Geometry: final body of the model. Coordinates: model frame, mm. A direction names the side the tool comes from. Give positions to 0.01 mm unless a question says otherwise; leave off trailing zeros. Write each loop counter-clockwise with the first axis right and the second up, starting at its lowest first coordinate (ties: lowest second). Pieces come first, ordered by that corner, then holes. Notation, with made-up numbers: M 73.5,18.25 L 109.5,18.25 A23 ccw 109.5,44.25 Z; hole C 5,-10.75 d6. An arc over 180 degrees is marked long. Answer as a JSON object with one key per item and string values.
from build123d import *

# Parameters (mm, degrees)
SKETCH_1_W          = 15.5
SKETCH_1_H          = 8
EXTRUDE_1_DEPTH     = 72
SKETCH_2_W          = 12.7
SKETCH_2_H          = 2
CUT_EXTRUDE_1_DEPTH = 75.082724032
SKETCH_3_W          = 15.5
SKETCH_3_H          = 4
EXTRUDE_2_DEPTH     = 2
SKETCH_5_R          = 2.1
CUT_EXTRUDE_3_DEPTH = 10


with BuildPart() as part:
    # 草图1 → 凸台-拉伸1 (new body)
    with BuildSketch(Plane.XY):
        with Locations((7.75, 4)):
            Rectangle(SKETCH_1_W, SKETCH_1_H)
    extrude(amount=EXTRUDE_1_DEPTH)

    # 草图2 → 切除-拉伸1 (cut, through all)
    with BuildSketch(Plane(origin=(0, 0, 0), x_dir=(-1, 0, 0), z_dir=(0, 0, -1))):
        with Locations((-7.75, 1)):
            Rectangle(SKETCH_2_W, SKETCH_2_H)
    extrude(amount=-CUT_EXTRUDE_1_DEPTH, mode=Mode.SUBTRACT)

    # 草图3 → 凸台-拉伸2 (add)
    with BuildSketch(Plane(origin=(0, 8, 0), x_dir=(1, 0, 0), z_dir=(0, 1, 0))):
        with Locations((7.75, -70)):
            Rectangle(SKETCH_3_W, SKETCH_3_H)
    extrude(amount=EXTRUDE_2_DEPTH)

    # 草图5 → 切除-拉伸3 (cut)
    with BuildSketch(Plane.XY.offset(72)):
        with Locations((3.75, 5)):
            Circle(SKETCH_5_R)
        with Locations(Location((11.75, 5, 0), (0, 0, 180))):
            Circle(SKETCH_5_R)
    extrude(amount=-CUT_EXTRUDE_3_DEPTH, mode=Mode.SUBTRACT)


solid = part.part
1) Pull-direction query (Y, two-part tool) for faces 1 (the flat face through (4, 5, 62)), 2 (the flat face through (15, 0, 35)), 3 (the flat face through (8, 10, 70)), 4 (the flat face through (1.4, 1, 35)); classes: pulls with the +Y half, pulls with the -Y half, needs draft (parallel to the pull), parting line crosses it, or undercut.
Geometry check:
{"face 1": "undercut", "face 2": "pulls with the -Y half", "face 3": "pulls with the +Y half", "face 4": "needs draft"}
2) Cut plane A-A on y = 5. Return loops of the section in (x, z), and give its area (3 significant figures).
Geometry check:
{"outline": "M 0,0 L 15.5,0 L 15.5,72 L 13.85,72 L 13.85,62 L 9.65,62 L 9.65,72 L 5.85,72 L 5.85,62 L 1.65,62 L 1.65,72 L 0,72 Z", "area": "1,030 mm2"}
3) Set-up query: faces 5 (the flat face through (8, 9, 68)), 6 (the cylindrical face through (4.88, 6.77, 67.07)), 7 (the flat face through (8, 5, 0)), 8 (the flat face through (14.1, 1, 35)). Return all of +Z, -Z, +X, -X, +Y, -Y with unobstructed straight access to the full face (end or side cutting, diameter ignored); none if empty.
Geometry check:
{"face 5": "-Z, +X, -X, +Y", "face 6": "+Z", "face 7": "-Z, +X, -X, +Y, -Y", "face 8": "+Z, -Z, -Y"}
4) Cut plane C-C on z = 40.5. Return loops of the section in (x, y).
Geometry check:
{"outline": "M 0,0 L 1.4,0 L 1.4,2 L 14.1,2 L 14.1,0 L 15.5,0 L 15.5,8 L 0,8 Z"}
5) Contact query for flat-ended pins moving along their axis: P1, Ø2, axis at x = 11, y = 5.5, coming from the +Z side; P2, Ø3.5, axis at x = 3.5, y = 5.5, coming from the +Z side; P3, Ø2, axis at x = 7, z = 60.5, coming from the +Y side; P4, Ø2, axis at x = 6, z = 23, coming from the -Y side. Output: stop coordinate, or through.
Geometry check:
{"P1": "stops at z = 62", "P2": "stops at z = 72", "P3": "stops at y = 8", "P4": "stops at y = 2"}
6) Line query: line 1 (Y direction, x = 3.75, z = 67.75); line 2 (X direction, y = 1.5, z = 10.5); line 3 (Y direction, x = 5, z = 27). Output: solid intervals per line, ascending. Write a range as from..to.
Geometry check:
{"line 1": "y = 2..2.9, 7.1..8", "line 2": "x = 0..1.4, 14.1..15.5", "line 3": "y = 2..8"}
7) Cut plane D-D on x = 3.75. Return loops of the section in (y, z).
Geometry check:
{"outline": "M 2,0 L 8,0 L 8,68 L 10,68 L 10,72 L 7.1,72 L 7.1,62 L 2.9,62 L 2.9,72 L 2,72 Z"}
8) Cut plane B-B on x = 9. Return loops of the section in (y, z).
Geometry check:
{"outline": "M 2,0 L 8,0 L 8,68 L 10,68 L 10,72 L 2,72 Z"}
